For this review, take the finished solid that the model builds, in its own axes (mm). Give positions to 0.01 mm unless a question says otherwise; leave off trailing zeros. Order: outer loops, then holes, each group sorted by start corner. A loop starts at its lowest first (then second) coordinate and runs counter-clockwise, first axis right, second up. Notation, with made-up numbers: (-22.5, 46.25) -> (14.5, 46.25) arc R21 ccw to (14.5, 68.25) -> close; hole circle Ø5 at (73.25, 37.5). An arc over 180 degrees is marked (long way). One line per item, written item: value. Start each with the question number.
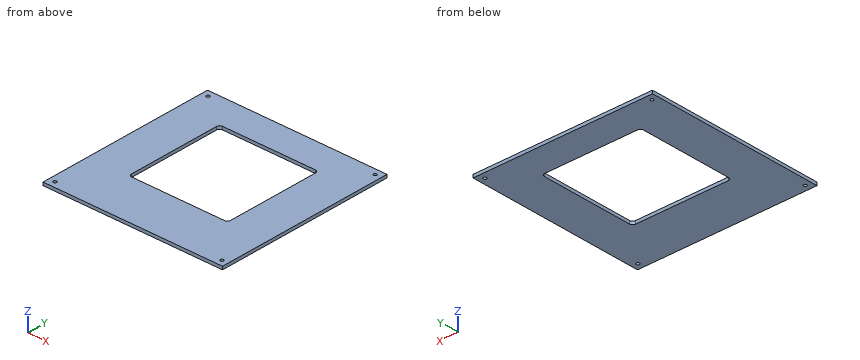
from build123d import *

# Parameters (mm, degrees)
F0_W     = 290
F0_H     = 290
F0_R     = 2.6
F1_DEPTH = 5
F3_DEPTH = 5.001


with BuildPart() as f1:
    # F0 (on Top) → F1 (new body)
    with BuildSketch(Plane.XY):
        Rectangle(F0_W, F0_H)
        with Locations((-135, -135)):
            Circle(F0_R, mode=Mode.SUBTRACT)
        with Locations((135, -135)):
            Circle(F0_R, mode=Mode.SUBTRACT)
        with Locations((-135, 135)):
            Circle(F0_R, mode=Mode.SUBTRACT)
        with Locations((135, 135)):
            Circle(F0_R, mode=Mode.SUBTRACT)
    extrude(amount=F1_DEPTH)

    # F2 (on face) → F3 (cut, through all)
    with BuildSketch(Plane.XY.offset(5)):
        with BuildLine():
            Line((-75, -65), (75, -65))
            ThreePointArc((75, -65), (78.535534, -63.535534), (80, -60))
            Line((80, -60), (80, 90))
            ThreePointArc((80, 90), (78.535534, 93.535534), (75, 95))
            Line((75, 95), (-75, 95))
            ThreePointArc((-75, 95), (-78.535534, 93.535534), (-80, 90))
            Line((-80, 90), (-80, -60))
            ThreePointArc((-80, -60), (-78.535534, -63.535534), (-75, -65))
        make_face()
    extrude(amount=-F3_DEPTH, mode=Mode.SUBTRACT)


solid = f1.part
Q1. Take a section at C-C (z = 2.4). State the section outline as (x, y) points, and give its area (3 significant figures).
Q2. For pin 1 Ø8.5 at (x, y) = (135, 135) entering from -Z, flat-tipped, find the tip position at first contact; note if it passes through.
Q3. For line 1 along Y through (x, z) = (135, 2.85); line 2 along X through (y, z) = (-7.5, 1.2), list the stretches that pass through material, from the lowest coordinate up.
Q4. Take a section at B-B (x = -46). State the section outline as (y, z) points, and give its area (3 significant figures).
Q5. Take a section at A-A (y = -45). State the section outline as (x, z) points, and give its area (3 significant figures).
Answers below:
1. outline: (-145, -145) -> (145, -145) -> (145, 145) -> (-145, 145) -> close; hole circle Ø5.2 at (-135, -135); hole circle Ø5.2 at (-135, 135); hole (-80, -60) arc R5 ccw to (-75, -65) -> (75, -65) arc R5 ccw to (80, -60) -> (80, 90) arc R5 ccw to (75, 95) -> (-75, 95) arc R5 ccw to (-80, 90) -> close; hole circle Ø5.2 at (135, -135); hole circle Ø5.2 at (135, 135)
1. area: 58,400 mm²
2. pin 1: stops at z = 0
3. line 1: y = -145 to -137.6, -132.4 to 132.4, 137.6 to 145
3. line 2: x = -145 to -80, 80 to 145
4. outline: (-145, 0) -> (-65, 0) -> (-65, 5) -> (-145, 5) -> close; (95, 0) -> (145, 0) -> (145, 5) -> (95, 5) -> close
4. area: 650 mm²
5. outline: (-145, 0) -> (-80, 0) -> (-80, 5) -> (-145, 5) -> close; (80, 0) -> (145, 0) -> (145, 5) -> (80, 5) -> close
5. area: 650 mm²
